Here's how the part is built. I have some questions about the finished solid (model axes, mm). Coordinates: 2 decimals unless noted, no trailing zeros. Write each loop counter-clockwise with the first axis right and the second up, starting at its lowest first coordinate (ties: lowest second). Pieces come first, ordered by that corner, then holes. Notation, with made-up numbers: M 60.25,28 L 90.25,28 A10 ccw 90.25,45 Z; hole C 3.5,-24 d3. An arc over 180 degrees is marked long. Use a Markdown table: item, result.
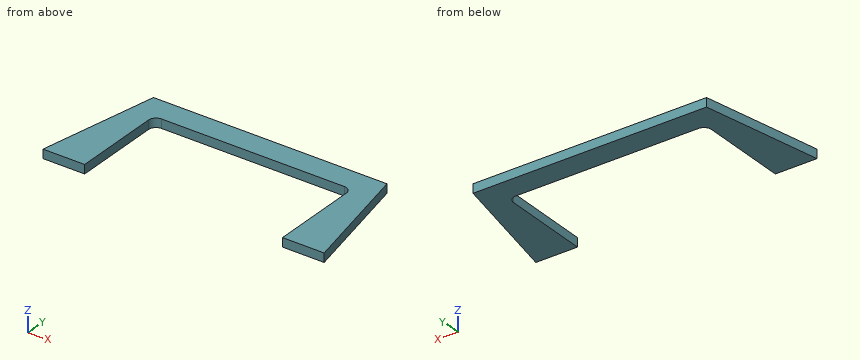
```python
from build123d import *

# Parameters (mm, degrees)
RESSALTO_EXTRUS_O1_DEPTH = 6


with BuildPart() as part:
    # Esboço1 → Ressalto-extrusão1 (new body)
    with BuildSketch(Plane.XY):
        with BuildLine():
            Line((-66.5, -40), (-94.5, -40))
            Line((-94.5, -40), (-78.5, 40))
            Line((-78.5, 40), (78.5, 40))
            Line((78.5, 40), (94.5, -40))
            Line((94.5, -40), (66.5, -40))
            Line((66.5, -40), (66.5, 19))
            ThreePointArc((66.5, 19), (65.035533906, 22.535533906), (61.5, 24))
            Line((61.5, 24), (-61.5, 24))
            ThreePointArc((-61.5, 24), (-65.035533906, 22.535533906), (-66.5, 19))
            Line((-66.5, 19), (-66.5, -40))
        make_face()
    extrude(amount=RESSALTO_EXTRUS_O1_DEPTH)


solid = part.part
```
1. Suppose I cut it at B-B on z = 1.25. Write out the boundary of the cut face in (x, y), and give its area (3 significant figures).
Answers follow:
| item | result |
|---|---|
| outline | M -94.5,-40 L -66.5,-40 L -66.5,19 A5 cw -61.5,24 L 61.5,24 A5 cw 66.5,19 L 66.5,-40 L 94.5,-40 L 78.5,40 L -78.5,40 Z |
| area | 5,340 mm2 |
2. I need wall thicknesses on probe 1 along Y at (x, z) = (5, 0.45); probe 2 along X at (y, z) = (21, 3.65); probe 3 along X at (y, z) = (16, 1.2). Which ranges of each line are inside material? Lowest first, please.
Answers follow:
| item | result |
|---|---|
| probe 1 | y = 24 to 40 |
| probe 2 | x = -82.3 to -66.08, 66.08 to 82.3 |
| probe 3 | x = -83.3 to -66.5, 66.5 to 83.3 |
3. Suppose I cut it at C-C on y = 9.5. Write out the boundary of the cut face in (x, z), and give its area (3 significant figures).
Answers follow:
| item | result |
|---|---|
| outline | M -84.6,0 L -66.5,0 L -66.5,6 L -84.6,6 Z; M 66.5,0 L 84.6,0 L 84.6,6 L 66.5,6 Z |
| area | 217 mm2 |
4. Suppose I cut it at D-D on x = -34. Write out the boundary of the cut face in (y, z), and give its area (3 significant figures).
Answers follow:
| item | result |
|---|---|
| outline | M 24,0 L 40,0 L 40,6 L 24,6 Z |
| area | 96.0 mm2 |
5. Suppose I cut it at A-A on y = -27.5. Write out the boundary of the cut face in (x, z).
Answers follow:
| item | result |
|---|---|
| outline | M -92,0 L -66.5,0 L -66.5,6 L -92,6 Z; M 66.5,0 L 92,0 L 92,6 L 66.5,6 Z |
6. Will these pins go through, and if not, where does the flat tip stop? pin 1 Ø3 at (x, z) = (-26.5, 2.5) entering from -Y; pin 2 Ø1 at (y, z) = (-23.5, 3) entering from -X.
Answers follow:
| item | result |
|---|---|
| pin 1 | stops at y = 24 |
| pin 2 | stops at x = -91.3 |
